Design review of the part built by this model. Coordinates are the model's own, in mm. A direction names the side the tool comes from. Round coordinates to 2 decimals unless told otherwise and drop trailing zeros. Loops run counter-clockwise (first coordinate to the right, second up) from the corner with the lowest first, then second, coordinate; pieces in that order, holes last. Notation, with made-up numbers: (11, -31.75) - (55, -31.75) arc R26 ccw to (55, -8.75) - close; hole circle Ø9 at (38.5, 76). An arc over 180 degrees is marked (long way). One line per question, with ' | ' between items. Start each with the question number.
from build123d import *

# Parameters (mm, degrees)
F0_R     = 12.5
F0_R_2   = 5
F1_DEPTH = 60
F2_DEPTH = 25


with BuildPart() as f1:
    # F0 (on Top) → F1 (new body)
    with BuildSketch(Plane.XY):
        Circle(F0_R)
        Circle(F0_R_2, mode=Mode.SUBTRACT)
        Circle(F0_R_2)
    extrude(amount=-F1_DEPTH)

    # F0 (on Top) → F2 (cut)
    with BuildSketch(Plane.XY):
        Circle(F0_R_2)
    extrude(amount=-F2_DEPTH, mode=Mode.SUBTRACT)

    # F3: F1 across face


with BuildPart() as f1_1:
    add(f1.part)
    add(f1.part.mirror(Plane(origin=(0, 0, -60), x_dir=(1, 0, 0), z_dir=(0, 0, -1))))


solid = f1_1.part
1. To check wall thickness, follow line 1 along Y through (x, z) = (0, -12.5); line 2 along Z through (x, y) = (3, 1.5); line 3 along Y through (x, z) = (0.25, -45). State the ranges of each line that lie inside material, in increasing order.
2. The part is to be moulded in two halves that separate along X. For faces 1 (the face through (11.923, 3.755, -60.84)), 2 (the face through (-1.08, -4.88, -12.32)), 3 (the face through (-0.2, -5.4, -120)), say which applies: pulls with the +X half, pulls with the -X half, needs draft (parallel to the pull), parting line crosses it, or undercut.
3. Take a section at C-C, the plane z = -48. Give the boundary of the cut face in (x, y), then the cut area to 3 significant figures.
4. Take a section at D-D, the plane z = -109.5. Give the boundary of the cut face in (x, y), then the cut area to 3 significant figures.
5. Clearance check with flat-ended pins moving along their axes: P1, Ø3, axis at x = 2, y = 2, coming from the +Z side; P2, Ø6, axis at y = -1, z = -105.5, coming from the -X side; P3, Ø6, axis at x = 0, y = 0, coming from the -Z side; P4, Ø1.5, axis at x = -2.5, z = -104, coming from the -Y side. State where each tip first meets the part, or that it passes through.
6. Machinability: for faces 4 (the face through (0, 0, -95)), 5 (the face through (-0.2, -5.4, 0)), 6 (the face through (0, 0, -25)), which of the approach directions +Z, -Z, +X, -X, +Y, -Y give a long, thin tool a straight path to every point of the face, cutting with its end or side? Answer none if there is none.
7. Take a section at A-A, the plane y = 0. Give the boundary of the cut face in (x, z).
Answer list:
1) line 1: y = -12.5 to -5, 5 to 12.5 | line 2: z = -95 to -25 | line 3: y = -12.5 to 12.5
2) face 1: parting line crosses it | face 2: undercut | face 3: needs draft
3) outline: circle Ø25 at (0, 0) | area: 491 mm²
4) outline: circle Ø25 at (0, 0); hole circle Ø10 at (0, 0) | area: 412 mm²
5) P1: stops at z = -25 | P2: stops at x = -12.5 | P3: stops at z = -95 | P4: stops at y = -12.38
6) face 4: -Z | face 5: +Z, +X, -X, +Y, -Y | face 6: +Z
7) outline: (-12.5, -120) - (-5, -120) - (-5, -95) - (5, -95) - (5, -120) - (12.5, -120) - (12.5, 0) - (5, 0) - (5, -25) - (-5, -25) - (-5, 0) - (-12.5, 0) - close
